Design review of the part built by this model. Coordinates are the model's own, in mm. A direction names the side the tool comes from. Give positions to 0.01 mm unless a question says otherwise; leave off trailing zeros. Loops run counter-clockwise (first coordinate to the right, second up) from the corner with the lowest first, then second, coordinate; pieces in that order, holes last. Notation, with made-up numbers: M 47,77.5 L 98,77.5 A21 cw 98,112.5 Z; hole C 75,-17 d2. An arc over 180 degrees is marked long. Answer as CSV lines item,"result".
```python
from build123d import *

# Parameters (mm, degrees)
CROQUIS1_R              = 3
SALIENTE_EXTRUIR1_DEPTH = 4
CROQUIS2_R              = 1.7
CORTAR_EXTRUIR1_DEPTH   = 4
CROQUIS3_R              = 2.95
CORTAR_EXTRUIR2_DEPTH   = 3


with BuildPart() as part:
    # Croquis1 → Saliente-Extruir1 (new body)
    with BuildSketch(Plane.XY):
        with BuildLine():
            Line((-7.200520814, 3.25), (-15, 3.25))
            Line((-15, 3.25), (-15, -3.25))
            Line((-15, -3.25), (-7.200520814, -3.25))
            ThreePointArc((-7.200520814, -3.25), (0, -7.9), (7.200520814, -3.25))
            Line((7.200520814, -3.25), (15, -3.25))
            Line((15, -3.25), (15, 3.25))
            Line((15, 3.25), (7.200520814, 3.25))
            ThreePointArc((7.200520814, 3.25), (0, 7.9), (-7.200520814, 3.25))
        make_face()
        Circle(CROQUIS1_R, mode=Mode.SUBTRACT)
    extrude(amount=SALIENTE_EXTRUIR1_DEPTH)

    # Croquis2 → Cortar-Extruir1 (cut)
    with BuildSketch(Plane.XY.offset(4)):
        with Locations((-11, 0)):
            Circle(CROQUIS2_R)
        with Locations((11, 0)):
            Circle(CROQUIS2_R)
    extrude(amount=-CORTAR_EXTRUIR1_DEPTH, mode=Mode.SUBTRACT)

    # Croquis3 → Cortar-Extruir2 (cut)
    with BuildSketch(Plane.XY.offset(4)):
        with Locations((-11, 0)):
            Circle(CROQUIS3_R)
        with Locations((11, 0)):
            Circle(CROQUIS3_R)
    extrude(amount=-CORTAR_EXTRUIR2_DEPTH, mode=Mode.SUBTRACT)


solid = part.part
```
1. The part is to be moulded in two halves that separate along Y. For faces 1 (the flat face through (11, -3.25, 2)), 2 (the flat face through (-0.2, -3.4, 0)), 3 (the flat face through (-11, -2, 1)), say which applies: pulls with the +Y half, pulls with the -Y half, needs draft (parallel to the pull), parting line crosses it, or undercut.
Answer block:
face 1,"pulls with the -Y half"
face 2,"needs draft"
face 3,"undercut"
2. We need section A-A, the plane x = 0. Write out the cut boundary in (y, z), plus the area to 3 significant figures.
Answer block:
outline,"M -7.9,0 L -3,0 L -3,4 L -7.9,4 Z; M 3,0 L 7.9,0 L 7.9,4 L 3,4 Z"
area,"39.2 mm²"
3. For faces 4 (the cylindrical face through (8.053, 0.13, 2.521)), 5 (the flat face through (-11, 3.25, 2)), 6 (the flat face through (-11, -3.25, 2)), list the 3-axis set-ups (+Z, -Z, +X, -X, +Y, -Y) from which the entire face can be reached by the end or side of a thin tool; tool diameter is ignored.
Answer block:
face 4,"+Z"
face 5,"+Z, -Z, -X, +Y"
face 6,"+Z, -Z, -X, -Y"
4. To check wall thickness, follow L1, parallel to X at y = 0.25, z = 2.95; L2, parallel to Y at x = 0, z = 2.75; L3, parallel to X at y = -1, z = 1.95. State the ranges of each line that lie inside material, in increasing order. Write a range as [from, to].
Answer block:
L1,"[-15, -13.94], [-8.06, -2.99], [2.99, 8.06], [13.94, 15]"
L2,"[-7.9, -3], [3, 7.9]"
L3,"[-15, -13.78], [-8.22, -2.83], [2.83, 8.22], [13.78, 15]"
5. We need section D-D, the plane z = 0.5. Write out the cut boundary in (x, y), plus the area to 3 significant figures.
Answer block:
outline,"M -15,-3.25 L -7.2,-3.25 A7.9 ccw 7.2,-3.25 L 15,-3.25 L 15,3.25 L 7.2,3.25 A7.9 ccw -7.2,3.25 L -15,3.25 Z; hole C -11,0 d3.4; hole C 0,0 d6; hole C 11,0 d3.4"
area,"245 mm²"
6. We need section C-C, the plane z = 3.7. Write out the cut boundary in (x, y).
Answer block:
outline,"M -15,-3.25 L -7.2,-3.25 A7.9 ccw 7.2,-3.25 L 15,-3.25 L 15,3.25 L 7.2,3.25 A7.9 ccw -7.2,3.25 L -15,3.25 Z; hole C -11,0 d5.9; hole C 0,0 d6; hole C 11,0 d5.9"
7. For P1, Ø1.5, axis at x = 5, z = 2.5, coming from the +Y side; P2, Ø2, axis at x = -12.5, z = 1.5, coming from the +Y side; P3, Ø1.5, axis at y = 5, z = 1.5, coming from the +X side, all flat-tipped, find the tip position at first contact; note any pin that passes through.
Answer block:
P1,"y = 6.66"
P2,"y = 3.25"
P3,"x = 6.66"
8. We need section B-B, the plane y = 0. Write out the cut boundary in (x, z).
Answer block:
outline,"M -15,0 L -12.7,0 L -12.7,1 L -13.95,1 L -13.95,4 L -15,4 Z; M -9.3,0 L -3,0 L -3,4 L -8.05,4 L -8.05,1 L -9.3,1 Z; M 3,0 L 9.3,0 L 9.3,1 L 8.05,1 L 8.05,4 L 3,4 Z; M 12.7,0 L 15,0 L 15,4 L 13.95,4 L 13.95,1 L 12.7,1 Z"
